```python
from build123d import *

# Parameters (mm, degrees)
ESBO_O3_R                = 75
ESBO_O3_R_2              = 15.5
RESSALTO_EXTRUS_O2_DEPTH = 9
CORTE_EXTRUS_O1_REACH    = 11


with BuildPart() as part:
    # Esboço3 → Ressalto-extrusão2 (new body)
    with BuildSketch(Plane(origin=(0, 0, 0), x_dir=(1, 0, 0), z_dir=(0, 1, 0))):
        with Locations(Location((0, 0, 0), (0, 0, 270))):  # turned: the seam where the file's is
            Circle(ESBO_O3_R)
        with Locations(Location((0, 0, 0), (0, 0, 270))):  # turned: the seam where the file's is
            Circle(ESBO_O3_R_2, mode=Mode.SUBTRACT)
    extrude(amount=RESSALTO_EXTRUS_O2_DEPTH)

    # Esboço5 → Corte-extrusão1 (cut, up to next)
    with BuildSketch(Plane(origin=(0, 9, 0), x_dir=(1, 0, 0), z_dir=(0, 1, 0)), mode=Mode.PRIVATE) as corte_extrus_o1_sk1:
        with BuildLine():
            ThreePointArc((0, 75), (-2.251014098, 74.966211959), (-4.5, 74.864878281))
            Line((-4.5, 74.864878281), (-4.5, 61))
            Line((-4.5, 61), (4.5, 61))
            Line((4.5, 61), (4.5, 74.864878281))
            ThreePointArc((4.5, 74.864878281), (2.251014098, 74.966211959), (0, 75))
        make_face()
    corte_extrus_o1_tool1 = extrude(corte_extrus_o1_sk1.sketch, amount=-CORTE_EXTRUS_O1_REACH, mode=Mode.PRIVATE) & part.part
    add(corte_extrus_o1_tool1.solids().sort_by_distance((0, 9, -67.977546))[0], mode=Mode.SUBTRACT)
    # Esboço5 → Corte-extrusão1 (cut, up to next)
    with BuildSketch(Plane(origin=(0, 9, 0), x_dir=(1, 0, 0), z_dir=(0, 1, 0)), mode=Mode.PRIVATE) as corte_extrus_o1_sk2:
        with BuildLine():
            Line((61, -4.5), (74.864878281, -4.5))
            ThreePointArc((74.864878281, -4.5), (74.966211959, -2.251014098), (75, 0))
            ThreePointArc((75, 0), (74.966211959, 2.251014098), (74.864878281, 4.5))
            Line((74.864878281, 4.5), (61, 4.5))
            Line((61, 4.5), (61, -4.5))
        make_face()
    corte_extrus_o1_tool2 = extrude(corte_extrus_o1_sk2.sketch, amount=-CORTE_EXTRUS_O1_REACH, mode=Mode.PRIVATE) & part.part
    add(corte_extrus_o1_tool2.solids().sort_by_distance((67.977546, 9, 0))[0], mode=Mode.SUBTRACT)
    # Esboço5 → Corte-extrusão1 (cut, up to next)
    with BuildSketch(Plane(origin=(0, 9, 0), x_dir=(1, 0, 0), z_dir=(0, 1, 0)), mode=Mode.PRIVATE) as corte_extrus_o1_sk3:
        with BuildLine():
            Line((-4.5, -61), (-4.5, -74.864878281))
            ThreePointArc((-4.5, -74.864878281), (-2.251014098, -74.966211959), (0, -75))
            ThreePointArc((0, -75), (2.251014098, -74.966211959), (4.5, -74.864878281))
            Line((4.5, -74.864878281), (4.5, -61))
            Line((4.5, -61), (-4.5, -61))
        make_face()
    corte_extrus_o1_tool3 = extrude(corte_extrus_o1_sk3.sketch, amount=-CORTE_EXTRUS_O1_REACH, mode=Mode.PRIVATE) & part.part
    add(corte_extrus_o1_tool3.solids().sort_by_distance((0, 9, 67.977546))[0], mode=Mode.SUBTRACT)
    # Esboço5 → Corte-extrusão1 (cut, up to next)
    with BuildSketch(Plane(origin=(0, 9, 0), x_dir=(1, 0, 0), z_dir=(0, 1, 0)), mode=Mode.PRIVATE) as corte_extrus_o1_sk4:
        with BuildLine():
            ThreePointArc((-75, 0), (-74.966211959, -2.251014098), (-74.864878281, -4.5))
            Line((-74.864878281, -4.5), (-61, -4.5))
            Line((-61, -4.5), (-61, 4.5))
            Line((-61, 4.5), (-74.864878281, 4.5))
            ThreePointArc((-74.864878281, 4.5), (-74.966211959, 2.251014098), (-75, 0))
        make_face()
    corte_extrus_o1_tool4 = extrude(corte_extrus_o1_sk4.sketch, amount=-CORTE_EXTRUS_O1_REACH, mode=Mode.PRIVATE) & part.part
    add(corte_extrus_o1_tool4.solids().sort_by_distance((-67.977546, 9, 0))[0], mode=Mode.SUBTRACT)


solid = part.part
```
Source: CAD feature listing. Evaluate the final solid. Frame: model axes, mm. A direction names the side the tool comes from. Coordinates: 2 decimals unless noted, no trailing zeros. Order: outer loops, then holes, each group sorted by start corner. A loop starts at its lowest first (then second) coordinate and runs counter-clockwise, first axis right, second up. Notation, with made-up numbers: M -27.75,57 L -14.75,57 A20 ccw -14.75,83 Z; hole C 51.5,-34.75 d10. An arc over 180 degrees is marked long. Write each question's results on one line, items separated by ' | '. Start each with the question number.
1) Section query D-D (x = 51.5). Return the cut outline in (y, z), plus the area to 3 significant figures.
2) Contact query for flat-ended pins moving along their axis: pin 1 Ø1.5 at (x, y) = (-19, 2.5) entering from -Z; pin 2 Ø4.5 at (x, y) = (0, 6) entering from +Z; pin 3 Ø2.5 at (x, y) = (-1.5, 4) entering from -Z. Output: stop coordinate, or through.
3) Section query B-B (x = 0). Return the cut outline in (y, z), plus the area to 3 significant figures.
4) Draft query along X for faces 1 (the face through (61, 5, 0)), 2 (the face through (15.368, 4.437, -2.018)), 3 (the face through (1, 9, 16)). Return one class per face: released by +X, released by -X, zero draft, split by the parting line, or undercut.
5) Section query A-A (z = 0). Return the cut outline in (x, y).
6) Access query for faces 4 (the face through (-68, 5, -4.5)), 5 (the face through (-4.5, 5, 68)), 6 (the face through (0, 5, -61)), 7 (the face through (68, 5, -4.5)). Directions: +Z, -Z, +X, -X, +Y, -Y. A direction counts if a zero-diameter tool reaches every point of the face in a straight line with its end or side. Return the directions, or none.
7) Line query: line 1 (X direction, y = 5.5, z = 0); line 2 (X direction, y = 5.5, z = -2.5); line 3 (Z direction, x = 5.5, y = 5.5). Output: solid intervals per line, ascending. Write a range as from..to.
8) Section query C-C (y = 6). Return the cut outline in (x, z).
Answers:
1) outline: M 0,-54.52 L 9,-54.52 L 9,54.52 L 0,54.52 Z | area: 981 mm^2
2) pin 1: stops at z = -72.75 | pin 2: stops at z = 61 | pin 3: stops at z = -61
3) outline: M 0,-61 L 9,-61 L 9,-15.5 L 0,-15.5 Z; M 0,15.5 L 9,15.5 L 9,61 L 0,61 Z | area: 819 mm^2
4) face 1: released by +X | face 2: undercut | face 3: zero draft
5) outline: M -61,0 L -15.5,0 L -15.5,9 L -61,9 Z; M 15.5,0 L 61,0 L 61,9 L 15.5,9 Z
6) face 4: -X, +Y, -Y | face 5: +Z, +Y, -Y | face 6: -Z, +Y, -Y | face 7: +X, +Y, -Y
7) line 1: x = -61..-15.5, 15.5..61 | line 2: x = -61..-15.3, 15.3..61 | line 3: z = -74.8..-14.49, 14.49..74.8
8) outline: M -74.86,-4.5 A75 ccw -4.5,-74.86 L -4.5,-61 L 4.5,-61 L 4.5,-74.86 A75 ccw 74.86,-4.5 L 61,-4.5 L 61,4.5 L 74.86,4.5 A75 ccw 4.5,74.86 L 4.5,61 L -4.5,61 L -4.5,74.86 A75 ccw -74.86,4.5 L -61,4.5 L -61,-4.5 Z; hole C 0,0 d31
